```python
from build123d import *

# Parameters (mm, degrees)
F1_DEPTH = 1.5
F0_W     = 20
F0_H     = 20
F2_DEPTH = 3
F4_DEPTH = 12.5


with BuildPart() as f1:
    # F0 (on Top) → F1 (new body)
    with BuildSketch(Plane.XY):
        with BuildLine():
            Line((22.912878, 10), (27.5, 10))
            Line((27.5, 10), (47.5, 10))
            Line((47.5, 10), (47.5, 12.5))
            Line((47.5, 12.5), (27.5, 12.5))
            Line((27.5, 12.5), (24.494897, 12.5))
            ThreePointArc((24.494897, 12.5), (-27.5, 0), (24.494897, -12.5))
            Line((24.494897, -12.5), (27.5, -12.5))
            Line((27.5, -12.5), (47.5, -12.5))
            Line((47.5, -12.5), (47.5, -10))
            Line((47.5, -10), (27.5, -10))
            Line((27.5, -10), (22.912878, -10))
            ThreePointArc((22.912878, -10), (-25, 0), (22.912878, 10))
        make_face()
    extrude(amount=F1_DEPTH)

    # F0 (on Top) → F2 (join)
    with BuildSketch(Plane.XY):
        with BuildLine():
            Line((27.5, -10), (27.5, 10))
            Line((27.5, 10), (22.912878, 10))
            ThreePointArc((22.912878, 10), (-25, 0), (22.912878, -10))
            Line((22.912878, -10), (27.5, -10))
        make_face()
        with Locations((37.5, 0)):
            Rectangle(F0_W, F0_H)
    extrude(amount=F2_DEPTH)

    # F3 (on Front) → F4 (join, symmetric)
    with BuildSketch(Plane.XZ):
        Polygon((47.5, 3), (47.5, 0), (57.039392, 0), align=None)
    extrude(amount=F4_DEPTH, both=True)


solid = f1.part
```
Here's how the part is built. I have some questions about the finished solid (model axes, mm). A direction names the side the tool comes from. Round coordinates to 2 decimals unless told otherwise and drop trailing zeros. Write each loop counter-clockwise with the first axis right and the second up, starting at its lowest first coordinate (ties: lowest second). Pieces come first, ordered by that corner, then holes.
Q1. If we section it at C-C on y = 0: Write out the boundary of the cut face in (x, z), plus the area to 3 significant figures.
Q2. Please list where these lines run through material, in increasing order: probe 1 along Y at (x, z) = (29.5, 2.4); probe 2 along Y at (x, z) = (29.5, 0.1); probe 3 along X at (y, z) = (-15, 1.45).
Q3. If we mould it in two halves opening along X, with no side actions, what happens to faces 5 (the cylindrical face through (-27.48, 1.03, 0.74)), 6 (the flat face through (21, -14, 1.5)), 7 (the flat face through (3, 0, 3)), 8 (the flat face through (52.336, -0.175, 1.479))? For each: +X half, -X half, draft (parallel to the pull), parting line (faces both ways), or undercut.
Q4. If we section it at D-D on z = 0.9: Write out the boundary of the cut face in (x, y).
Q5. If we section it at B-B on y = 20.5: Write out the boundary of the cut face in (x, z).
Q6. Which directions (+Z, -Z, +X, -X, +Y, -Y) give clear straight access to the entire face, cutting with the end or side of a thin tool? Please do faces 1 (the flat face through (41, 12.5, 1)), 2 (the flat face through (41, -12.5, 1)), 3 (the cylindrical face through (-24.98, 0.96, 2.24)), 4 (the flat face through (5, 0, 0)).
Q7. Will these pins go through, and if not, where does the flat tip stop? P1, Ø1, axis at y = 14, z = 2.5, coming from the -X side; P2, Ø1.6, axis at y = -11, z = 2.5, coming from the -X side; P3, Ø0.8, axis at y = 11.5, z = 2, coming from the -X side; P4, Ø3, axis at x = 39, y = -13, coming from the -Z side.
Q8. If we section it at A-A on x = 0: Write out the boundary of the cut face in (y, z), plus the area to 4 significant figures.
Answer below:
1. outline: (-27.5, 0) - (57.04, 0) - (47.5, 3) - (-25, 3) - (-25, 1.5) - (-27.5, 1.5) - close
1. area: 236 mm2
2. probe 1: y = -10 to 10
2. probe 2: y = -12.5 to 12.5
2. probe 3: x = -23.05 to 23.05
3. face 5: parting line
3. face 6: undercut
3. face 7: draft
3. face 8: +X half
4. outline: (24.49, -12.5) - (54.18, -12.5) - (54.18, 12.5) - (24.49, 12.5) arc R27.5 ccw (long way) to start
5. outline: (-18.33, 0) - (18.33, 0) - (18.33, 1.5) - (14.31, 1.5) - (14.31, 3) - (-14.31, 3) - (-14.31, 1.5) - (-18.33, 1.5) - close
6. face 1: +Z, -Z, +X, +Y
6. face 2: +Z, -Z, +X, -Y
6. face 3: +Z
6. face 4: -Z, +X, -X, +Y, -Y
7. P1: stops at x = -21.04
7. P2: stops at x = -22.82
7. P3: stops at x = -22.4
7. P4: stops at z = 0
8. outline: (-27.5, 0) - (27.5, 0) - (27.5, 1.5) - (25, 1.5) - (25, 3) - (-25, 3) - (-25, 1.5) - (-27.5, 1.5) - close
8. area: 157.5 mm2
